```python
from build123d import *


with BuildPart() as part:
    # Sketch1 → Revolve1 (revolve)
    with BuildSketch(Plane(origin=(0, 0, 0), x_dir=(1, 0, 0), z_dir=(0, 1, 0))):
        with BuildLine():
            ThreePointArc((9.04875, 2.032), (9.281494477, 2.107409957), (9.425791706, 2.304982636))
            Line((9.425791706, 2.304982636), (10.033, 4.1529))
            Line((10.033, 4.1529), (11.6205, 4.1529))
            Line((11.6205, 4.1529), (11.6205, 2.5654))
            ThreePointArc((11.6205, 2.5654), (10.869111736, 0.751388264), (9.0551, 0))
            Line((9.0551, 0), (4.7625, 0))
            Line((4.7625, 0), (4.7625, 2.032))
            Line((4.7625, 2.032), (9.04875, 2.032))
        make_face()
    revolve(axis=Axis((0, 0, 0), (0, 0, -1)))


solid = part.part
```
CAD build for the part. Positions are in the model's coordinates, mm. Give positions to 0.01 mm unless a question says otherwise; leave off trailing zeros. Write each loop counter-clockwise with the first axis right and the second up, starting at its lowest first coordinate (ties: lowest second). Pieces come first, ordered by that corner, then holes. Notation, with made-up numbers: M 58,-33.5 L 74,-33.5 A24 ccw 74,-10.5 Z; hole C 36,-30 d9. An arc over 180 degrees is marked long. Return JSON: item names as keys, results as strings. Group by question number.
(1) Drill centre lines: L1, parallel to X at y = -4.25, z = -2; L2, parallel to Z at x = 5, y = 6.5; L3, parallel to X at y = 3.5, z = -0.7. Where is each one in solid material? Low to high. Write a range as [from, to].
(2) Band-saw the part on A-A (y = 0). Give the cut face in (x, z), and give its area (3 significant figures).
(3) Mould opens along Y. For faces 1 (the face through (5.36, 10.31, -3.35)), 2 (the face through (-4, 4, -2.032)), 3 (the face through (4, 4, 0)) say: pulls with the +Y half, pulls with the -Y half, needs draft (parallel to the pull), parting line crosses it, or undercut.
(4) Flat gauge pins, fed straight in: pin 1 Ø1 at (x, z) = (-9.5, -3.5) entering from -Y; pin 2 Ø5 at (x, y) = (-1, 3.5) entering from +Z; pin 3 Ø5.5 at (x, y) = (-2.5, -2.5) entering from -Z; pin 4 Ø1.5 at (y, z) = (-2, -0.5) entering from +X. Where does each tip first touch, or does it go through?
(5) Band-saw the part on D-D (z = -1.4). Give the cut face in (x, y) (1 decimal), and give its area (3 significant figures).
(6) Band-saw the part on C-C (z = -3.1). Give the cut face in (x, y).
Entries:
{
 "1": {"L1": "x = [-10.75, -2.15], [2.15, 10.75]", "L2": "z = [-2.03, 0]", "L3": "x = [-10.23, -3.23], [3.23, 10.23]"},
 "2": {"outline": "M -11.62,-4.15 L -10.03,-4.15 L -9.43,-2.3 A0.4 cw -9.05,-2.03 L -4.76,-2.03 L -4.76,0 L -9.06,0 A2.57 ccw -11.62,-2.57 Z; M 4.76,-2.03 L 9.05,-2.03 A0.4 cw 9.43,-2.3 L 10.03,-4.15 L 11.62,-4.15 L 11.62,-2.57 A2.57 ccw 9.06,0 L 4.76,0 Z", "area": "33.3 mm^2"},
 "3": {"face 1": "parting line crosses it", "face 2": "undercut", "face 3": "needs draft"},
 "4": {"pin 1": "stops at y = -7.35", "pin 2": "stops at z = 0", "pin 3": "stops at z = -2.03", "pin 4": "stops at x = 11.1"},
 "5": {"outline": "C 0,0 d22.7; hole C 0,0 d9.5", "area": "333 mm^2"},
 "6": {"outline": "C 0,0 d23.24; hole C 0,0 d19.37"}
}
